Source: three-view drawing plus pictorial views. Frame: mm from the lowest corner of the part. Coordinates: 2 decimals unless noted, no trailing zeros. Order: outer loops, then holes, each group sorted by start corner. A loop starts at its lowest first (then second) coordinate and runs counter-clockwise, first axis right, second up. Notation, with made-up numbers: (23.25, -13.75) - (73.25, -13.75) arc R30 ccw to (73.25, 25.25) - close; hole circle Ø6 at (12.25, 71). An arc over 180 degrees is marked (long way). One line per question, with ' | ' between items.
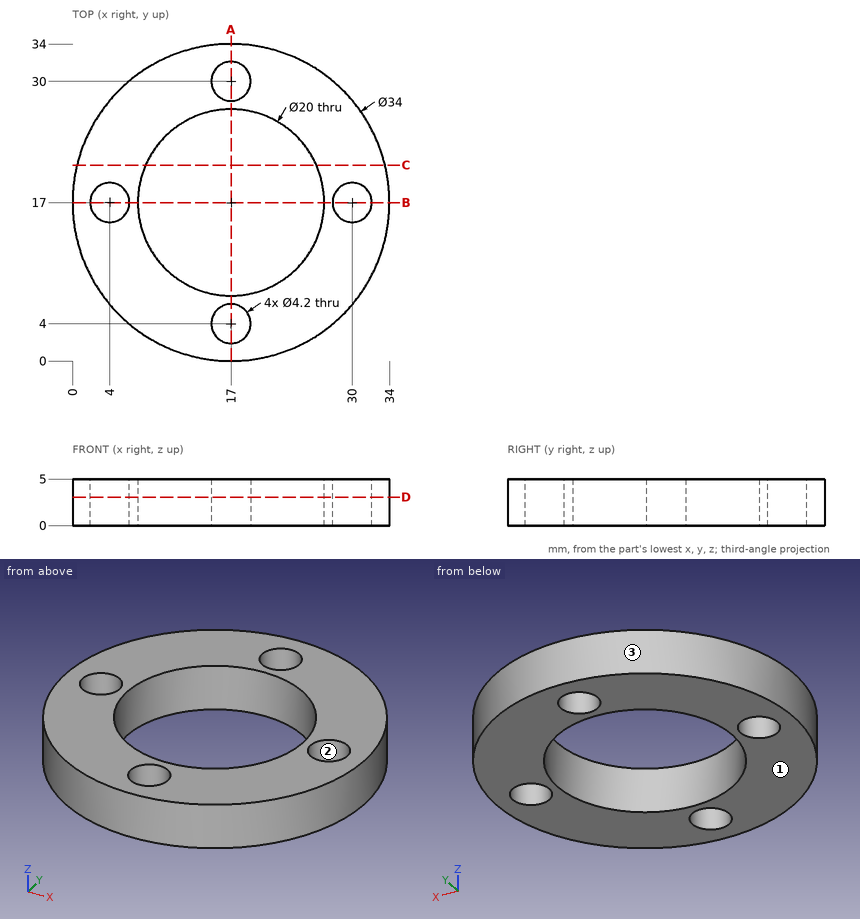
(1) Pin query (flat end, axial travel): P1, Ø3, axis at x = 23, z = 3, coming from the +Y side; P2, Ø1.5, axis at x = 6.5, z = 2.5, coming from the +Y side; P3, Ø2, axis at y = 17.5, z = 4.5, coming from the +X side. Return the tip coordinate at first contact, or that it passes through.
Taken from the geometry:
P1: stops at y = 33.39 | P2: stops at y = 30.93 | P3: stops at x = 34
(2) Pull-direction query (X, two-part tool) for the marked faces 1, 2 and 3; classes: pulls with the +X half, pulls with the -X half, needs draft (parallel to the pull), parting line crosses it, or undercut.
Taken from the geometry:
face 1: needs draft | face 2: undercut | face 3: parting line crosses it
(3) Cut plane D-D (z = 3.05). Return the cut outline in (x, y), and give its area (3 significant figures).
Taken from the geometry:
outline: circle Ø34 at (17, 17); hole circle Ø4.2 at (4, 17); hole circle Ø20 at (17, 17); hole circle Ø4.2 at (17, 4); hole circle Ø4.2 at (17, 30); hole circle Ø4.2 at (30, 17) | area: 538 mm²
(4) Cut plane C-C (y = 21). Return the cut outline in (x, z).
Taken from the geometry:
outline: (0.48, 0) - (7.83, 0) - (7.83, 5) - (0.48, 5) - close; (26.17, 0) - (33.52, 0) - (33.52, 5) - (26.17, 5) - close
(5) Cut plane A-A (x = 17). Return the cut outline in (y, z), and give its area (3 significant figures).
Taken from the geometry:
outline: (0, 0) - (1.9, 0) - (1.9, 5) - (0, 5) - close; (6.1, 0) - (7, 0) - (7, 5) - (6.1, 5) - close; (27, 0) - (27.9, 0) - (27.9, 5) - (27, 5) - close; (32.1, 0) - (34, 0) - (34, 5) - (32.1, 5) - close | area: 28.0 mm²
(6) Material intervals for L1, parallel to Y at x = 17, z = 3.1; L2, parallel to X at y = 16, z = 0.25; L3, parallel to Y at x = 8, z = 0.6, sorted ascending. Write a range as from..to.
Taken from the geometry:
L1: y = 0..1.9, 6.1..7, 27..27.9, 32.1..34 | L2: x = 0.03..2.15, 5.85..7.05, 26.95..28.15, 31.85..33.97 | L3: y = 2.58..12.64, 21.36..31.42
